Input: part model. Units: mm. Frame: model coordinates. A direction names the side the tool comes from. Give positions to 0.01 mm unless a question says otherwise; leave off trailing zeros. Loops run counter-clockwise (first coordinate to the right, second up) from the corner with the lowest first, then second, coordinate; pieces in that order, holes last. Notation, with made-up numbers: M 89.5,61.5 L 108.5,61.5 A21 ccw 108.5,100.5 Z; hole C 70,-33 d3. An arc over 180 degrees is marked long. One line per item, written item: value. Start each with the question number.
(1) Pin query (flat end, axial travel): P1, Ø3, axis at y = -2.5, z = 112, coming from the +X side; P2, Ø2, axis at x = 4, z = 133, coming from the +Y side; P3, Ø5, axis at x = 5.5, z = 187, coming from the -Y side. Return the tip coordinate at first contact, or that it passes through.
(2) Ray query, line 1 along Z through (x, y) = (4, -5); line 2 along Z through (x, y) = (4, 0.5); line 3 along X through (y, z) = (1, 328). Return the intervals inside material, ascending. Write a range as from..to.
(3) Access query for faces 1 (the flat face through (-4, 4, 369)), 2 (the cylindrical face through (5.723, -1.802, -3.451)), 3 (the cylindrical face through (-1.73, -7.81, 178.47)). Directions: +Z, -Z, +X, -X, +Y, -Y. A direction counts if a zero-diameter tool reaches every point of the face in a straight line with its end or side. Return the directions, or none.
(4) Section C-C on z = 27.5. Output: boundary loops of the cut face in (x, y).
```python
from build123d import *

# Parameters (mm, degrees)
SKETCH1_R           = 8
BOSS_EXTRUDE1_DEPTH = 362
SKETCH6_R           = 6
BOSS_EXTRUDE2_DEPTH = 5
SKETCH7_R           = 6
BOSS_EXTRUDE3_DEPTH = 2
SKETCH8_R           = 5
BOSS_EXTRUDE4_DEPTH = 10
SKETCH9_R           = 4
BOSS_EXTRUDE5_DEPTH = 10
CHAMFER1_SIZE       = 1
CHAMFER2_SIZE       = 1
BOSS_EXTRUDE6_START = 5
SKETCH10_R          = 6
BOSS_EXTRUDE6_DEPTH = 5
BOSS_EXTRUDE7_START = 2
SKETCH11_R          = 6
BOSS_EXTRUDE7_DEPTH = 2
BOSS_EXTRUDE8_START = 10
SKETCH12_R          = 5
BOSS_EXTRUDE8_DEPTH = 10
CHAMFER3_SIZE       = 1


with BuildPart() as part:
    # Sketch1 → Boss-Extrude1 (new body)
    with BuildSketch(Plane.XY):
        Circle(SKETCH1_R)
    extrude(amount=BOSS_EXTRUDE1_DEPTH)

    # Sketch6 → Boss-Extrude2 (add)
    with BuildSketch(Plane(origin=(0, 0, 0), x_dir=(-1, 0, 0), z_dir=(0, 0, -1))):
        with Locations(Location((0, 0, 0), (0, 0, 180))):
            Circle(SKETCH6_R)
    extrude(amount=BOSS_EXTRUDE2_DEPTH)

    # Sketch7 → Boss-Extrude3 (add)
    with BuildSketch(Plane(origin=(0, 0, -5), x_dir=(-1, 0, 0), z_dir=(0, 0, -1))):
        with Locations(Location((0, 0, 0), (0, 0, 180))):
            Circle(SKETCH7_R)
    extrude(amount=BOSS_EXTRUDE3_DEPTH)

    # Sketch8 → Boss-Extrude4 (add)
    with BuildSketch(Plane(origin=(0, 0, -7), x_dir=(-1, 0, 0), z_dir=(0, 0, -1))):
        Circle(SKETCH8_R)
    extrude(amount=BOSS_EXTRUDE4_DEPTH)

    # Sketch9 → Boss-Extrude5 (add)
    with BuildSketch(Plane(origin=(0, 0, -17), x_dir=(-1, 0, 0), z_dir=(0, 0, -1))):
        Circle(SKETCH9_R)
    extrude(amount=BOSS_EXTRUDE5_DEPTH)

    # Chamfer1
    chamfer1_edges = [part.edges().sort_by_distance(p)[0] for p in [
        (5, 0, -17),
    ]]
    chamfer(chamfer1_edges, length=CHAMFER1_SIZE - 0.0001)  # a hair under: the kernel refuses the full size

    # Chamfer2
    chamfer2_edges = [part.edges().sort_by_distance(p)[0] for p in [
        (4, 0, -27),
    ]]
    chamfer(chamfer2_edges, length=CHAMFER2_SIZE)

    # Sketch10 → Boss-Extrude6 (add)
    with BuildSketch(Plane.XY.offset(362).offset(BOSS_EXTRUDE6_START)):
        Circle(SKETCH10_R)
    extrude(amount=-BOSS_EXTRUDE6_DEPTH)

    # Sketch11 → Boss-Extrude7 (add)
    with BuildSketch(Plane.XY.offset(367).offset(BOSS_EXTRUDE7_START)):
        Circle(SKETCH11_R)
    extrude(amount=-BOSS_EXTRUDE7_DEPTH)

    # Sketch12 → Boss-Extrude8 (add)
    with BuildSketch(Plane.XY.offset(369).offset(BOSS_EXTRUDE8_START)):
        with Locations(Location((0, 0, 0), (0, 0, 180))):
            Circle(SKETCH12_R)
    extrude(amount=-BOSS_EXTRUDE8_DEPTH)

    # Chamfer3
    chamfer3_edges = [part.edges().sort_by_distance(p)[0] for p in [
        (5, 0, 379),
    ]]
    chamfer(chamfer3_edges, length=CHAMFER3_SIZE)


solid = part.part
```
Output values:
1. P1: stops at x = 7.94
1. P2: stops at y = 7.42
1. P3: stops at y = -7.42
2. line 1: z = 0..362
2. line 2: z = -16.97..378.97
2. line 3: x = -7.94..7.94
3. face 1: +Z
3. face 2: -Z
3. face 3: +Z, -Z
4. outline: C 0,0 d16
